```python
from build123d import *

# Parameters (mm, degrees)
BOSS_EXTRUDE1_DEPTH = 10
BOSS_EXTRUDE2_DEPTH = 16


with BuildPart() as part:
    # Sketch1 → Boss-Extrude1 (new body)
    with BuildSketch(Plane(origin=(0, 0, 0), x_dir=(0, 0, -1), z_dir=(1, 0, 0))):
        Polygon((-19.511221689, 9.49340082), (-14.056806101, 9.49340082), (-11.484013895, 12.066193026), (-11.484013895, 13.49340082), (-13.684013895, 13.49340082), (-19.884013895, 13.49340082), (-22.084013895, 13.49340082), (-22.084013895, 12.066193026), align=None)
    extrude(amount=BOSS_EXTRUDE1_DEPTH)

    # Sketch2 → Boss-Extrude2 (add)
    with BuildSketch(Plane(origin=(0, 13.49340082, 0), x_dir=(1, 0, 0), z_dir=(0, 1, 0))):
        with BuildLine():
            ThreePointArc((7.5, -16.784013895), (6.767766953, -15.016246942), (5, -14.284013895))
            Line((5, -14.284013895), (5, -16.784013895))
            Line((5, -16.784013895), (7.5, -16.784013895))
        make_face()
        with BuildLine():
            Line((5, -16.784013895), (5, -14.284013895))
            ThreePointArc((5, -14.284013895), (3.232233047, -15.016246942), (2.5, -16.784013895))
            Line((2.5, -16.784013895), (5, -16.784013895))
        make_face()
        with BuildLine():
            Line((7.5, -16.784013895), (5, -16.784013895))
            Line((5, -16.784013895), (5, -19.284013895))
            ThreePointArc((5, -19.284013895), (6.767766953, -18.551780848), (7.5, -16.784013895))
        make_face()
        with BuildLine():
            Line((5, -19.284013895), (5, -16.784013895))
            Line((5, -16.784013895), (2.5, -16.784013895))
            ThreePointArc((2.5, -16.784013895), (3.232233047, -18.551780848), (5, -19.284013895))
        make_face()
    extrude(amount=BOSS_EXTRUDE2_DEPTH)


solid = part.part
```
Here's how the part is built. I have some questions about the finished solid (model axes, mm). A direction names the side the tool comes from. Round coordinates to 2 decimals unless told otherwise and drop trailing zeros. Write each loop counter-clockwise with the first axis right and the second up, starting at its lowest first coordinate (ties: lowest second). Pieces come first, ordered by that corner, then holes.
Q1. If we section it at D-D on x = 7.25: Write out the boundary of the cut face in (y, z).
Q2. If we section it at C-C on y = 18.5: Write out the boundary of the cut face in (x, z).
Q3. Please list where these lines run through material, in increasing order: probe 1 along Y at (x, z) = (2, 19.5); probe 2 along X at (y, z) = (23.75, 16.5); probe 3 along X at (y, z) = (27.75, 15.5).
Q4. Which directions (+Z, -Z, +X, -X, +Y, -Y) give clear straight access to the entire face, cutting with the end or side of a thin tool? Please do faces 1 (the flat face through (0, 12, 17)), 2 (the flat face through (4, 13.493, 14)).
Q5. If we section it at B-B on z = 18.5: Write out the boundary of the cut face in (x, y), plus the area to 3 significant figures.
Q6. Will these pins go through, and if not, where does the flat tip stop? P1, Ø3, axis at x = 2, z = 16, coming from the +Y side; P2, Ø4, axis at y = 26, z = 19, coming from the -X side; P3, Ø1, axis at x = 7.5, z = 13, coming from the -Y side; P4, Ø6, axis at y = 21, z = 13, coming from the -X side.
Q7. If we section it at A-A on x = 8.5: Write out the boundary of the cut face in (y, z).
Answer below:
1. outline: (9.49, 14.06) - (12.07, 11.48) - (13.49, 11.48) - (13.49, 15.69) - (29.49, 15.69) - (29.49, 17.87) - (13.49, 17.87) - (13.49, 22.08) - (12.07, 22.08) - (9.49, 19.51) - close
2. outline: circle Ø5 at (5, 16.78)
3. probe 1: y = 9.49 to 13.49
3. probe 2: x = 2.52 to 7.48
3. probe 3: x = 2.85 to 7.15
4. face 1: +Z, -Z, -X, +Y, -Y
4. face 2: +Y
5. outline: (0, 9.49) - (10, 9.49) - (10, 13.49) - (6.82, 13.49) - (6.82, 29.49) - (3.18, 29.49) - (3.18, 13.49) - (0, 13.49) - close
5. area: 98.2 mm2
6. P1: stops at y = 29.49
6. P2: stops at x = 2.51
6. P3: stops at y = 10.05
6. P4: stops at x = 2.63
7. outline: (9.49, 14.06) - (12.07, 11.48) - (13.49, 11.48) - (13.49, 22.08) - (12.07, 22.08) - (9.49, 19.51) - close
